Here's how the part is built. I have some questions about the finished solid (model axes, mm). Give positions to 0.01 mm unless a question says otherwise; leave off trailing zeros. Write each loop counter-clockwise with the first axis right and the second up, starting at its lowest first coordinate (ties: lowest second). Pieces come first, ordered by that corner, then holes. Notation, with made-up numbers: (8, 11) -> (56, 11) arc R13 ccw to (56, 22) -> close; hole circle Ø4 at (-14.75, 24). An arc over 180 degrees is marked (long way). Return JSON: item names as keys, results as strings.
from build123d import *

# Parameters (mm, degrees)
SKETCH1_R           = 47
SKETCH1_R_2         = 1.3
SKETCH1_R_3         = 15
SKETCH1_R_4         = 1.25
BOSS_EXTRUDE1_DEPTH = 5


with BuildPart() as part:
    # Sketch1 → Boss-Extrude1 (new body)
    with BuildSketch(Plane.XY):
        Circle(SKETCH1_R)
        with Locations((0, 43.5)):
            Circle(SKETCH1_R_2, mode=Mode.SUBTRACT)
        with Locations((43.5, 0)):
            Circle(SKETCH1_R_2, mode=Mode.SUBTRACT)
        with Locations((0, -43.5)):
            Circle(SKETCH1_R_2, mode=Mode.SUBTRACT)
        with Locations((-43.5, 0)):
            Circle(SKETCH1_R_2, mode=Mode.SUBTRACT)
        Circle(SKETCH1_R_3, mode=Mode.SUBTRACT)
        with Locations((-19.798989873, 19.798989873)):
            Circle(SKETCH1_R_4, mode=Mode.SUBTRACT)
        with Locations((19.798989873, 19.798989873)):
            Circle(SKETCH1_R_4, mode=Mode.SUBTRACT)
        with Locations((19.798989873, -19.798989873)):
            Circle(SKETCH1_R_4, mode=Mode.SUBTRACT)
        with Locations((-19.798989873, -19.798989873)):
            Circle(SKETCH1_R_4, mode=Mode.SUBTRACT)
    extrude(amount=BOSS_EXTRUDE1_DEPTH)


solid = part.part
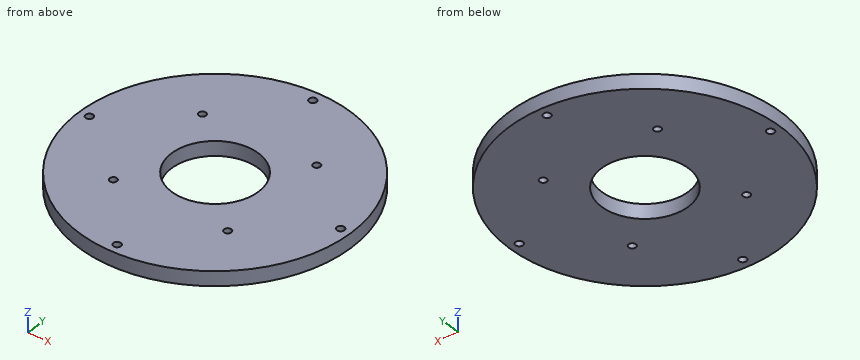
1. For pin 1 Ø3 at (y, z) = (-8, 4) entering from +X; pin 2 Ø2 at (x, z) = (7.5, 3.5) entering from -Y; pin 3 Ø1.5 at (y, z) = (-14.5, 2) entering from +X, each with a flat end and sliding along its axis, tell me the tip position at first contact or that it passes through.
Taken from the geometry:
{"pin 1": "stops at x = 46.55", "pin 2": "stops at y = -46.55", "pin 3": "stops at x = 44.94"}
2. Suppose I cut it at D-D, the plane z = 1.1. Count the separate pieces of the cut face and the enclosed holes in it, and give its area (3 significant figures).
Taken from the geometry:
{"separate pieces": "1", "enclosed holes": "9", "area": "6,190 mm²"}
3. Suppose I cut it at C-C, the plane x = -43.5. List the corners of the cut face in (y, z) for me.
Taken from the geometry:
{"outline": "(-17.8, 0) -> (-1.3, 0) -> (-1.3, 5) -> (-17.8, 5) -> close; (1.3, 0) -> (17.8, 0) -> (17.8, 5) -> (1.3, 5) -> close"}
4. Suppose I cut it at A-A, the plane x = 0. List the corners of the cut face in (y, z) for me.
Taken from the geometry:
{"outline": "(-47, 0) -> (-44.8, 0) -> (-44.8, 5) -> (-47, 5) -> close; (-42.2, 0) -> (-15, 0) -> (-15, 5) -> (-42.2, 5) -> close; (15, 0) -> (42.2, 0) -> (42.2, 5) -> (15, 5) -> close; (44.8, 0) -> (47, 0) -> (47, 5) -> (44.8, 5) -> close"}
5. If I drill on line 1 (Y direction, x = 0, z = 1.65); line 2 (X direction, y = -19.5, z = 1.25); line 3 (X direction, y = 20, z = 2.9), over which ranges is the centre line in solid material (lowest first)? Write a range as [from, to].
Taken from the geometry:
{"line 1": "y = [-47, -44.8], [-42.2, -15], [15, 42.2], [44.8, 47]", "line 2": "x = [-42.76, -21.01], [-18.59, 18.59], [21.01, 42.76]", "line 3": "x = [-42.53, -21.03], [-18.57, 18.57], [21.03, 42.53]"}
